Read the model definition and answer for the solid it produces. Units are mm, in the model's axes. A direction names the side the tool comes from. Coordinates: 2 decimals unless noted, no trailing zeros. Order: outer loops, then holes, each group sorted by start corner. A loop starts at its lowest first (then second) coordinate and runs counter-clockwise, first axis right, second up. Notation, with made-up numbers: (8.25, 27.5) - (58.25, 27.5) arc R8 ccw to (58.25, 34.5) - close; hole circle Ø8 at (38.5, -27.75). An arc over 180 degrees is marked (long way). Use one line per item in the form item = value.
```python
from build123d import *

# Parameters (mm, degrees)
F0_R     = 26.745197
F1_DEPTH = 50.8
F2_R     = 33.58545
F3_DEPTH = 101.6
F4_DEPTH = 50.8
F5_DEPTH = 25.4
F6_W     = 15.942245
F6_H     = 27.044877
F7_DEPTH = 152.4


with BuildPart() as f1:
    # F0 (on Top) → F1 (new body)
    with BuildSketch(Plane.XY):
        with Locations((-60.452543, 36.618207)):
            Circle(F0_R)
    extrude(amount=F1_DEPTH)

    # F2 (on Top) → F3 (join)
    with BuildSketch(Plane.XY):
        with Locations((-27.838308, 13.809561)):
            Circle(F2_R)
    extrude(amount=F3_DEPTH)

    # F0 (on Top) → F4 (join)
    with BuildSketch(Plane.XY):
        with Locations((-60.452543, 36.618207)):
            Circle(F0_R)
    extrude(amount=F4_DEPTH)

    # F0 (on Top) → F5 (join)
    with BuildSketch(Plane.XY):
        with Locations((-60.452543, 36.618207)):
            Circle(F0_R)
    extrude(amount=-F5_DEPTH)

    # F6 (on Top) → F7 (join)
    with BuildSketch(Plane.XY):
        with Locations((-24.767418, 13.522438)):
            Rectangle(F6_W, F6_H)
    extrude(amount=-F7_DEPTH)


solid = f1.part
```
(1) Section D-D, the plane y = -8 is taken. Write down the section's boundary in (x, z).
Answer list:
outline = (-53.38, 0) - (-2.3, 0) - (-2.3, 101.6) - (-53.38, 101.6) - close
(2) Section B-B, the plane x = -21 is taken. Write down the section's boundary in (y, z), then the cut area to 3 significant figures.
Answer list:
outline = (-19.07, 0) - (0, 0) - (0, -152.4) - (27.04, -152.4) - (27.04, 0) - (46.69, 0) - (46.69, 101.6) - (-19.07, 101.6) - close
area = 10,800 mm2
(3) Given pin 1 Ø12 at (x, y) = (-33.5, -6.5) entering from -Z; pin 2 Ø1 at (x, y) = (-69.5, 15.5) entering from -Z; pin 3 Ø13.5 at (y, z) = (19.5, -85) entering from -X, each flat-ended and moving along its own axis, determine where each tip first touches the part or whether it passes through.
Answer list:
pin_1 = 0
pin_2 = -25.4
pin_3 = -32.74
(4) Section A-A, the plane z = -68 is taken. Write down the section's boundary in (x, y).
Answer list:
outline = (-32.74, 0) - (-16.8, 0) - (-16.8, 27.04) - (-32.74, 27.04) - close
(5) Straight lines are drawn through the part: L1, parallel to Z at x = -79.5, y = 23; L2, parallel to Z at x = -2, y = 18; L3, parallel to X at y = 10.5, z = -88. For each, find the intervals that lie inside material, in ascending order.
Answer list:
L1 = -25.4 to 50.8
L2 = 0 to 101.6
L3 = -32.74 to -16.8
(6) Which of the six approach directions +Z, -Z, +X, -X, +Y, -Y give full straight-line access (tool end or side, diameter ignored) to faces 1 (the flat face through (-25, 27.045, -75)), 2 (the flat face through (-25, 0, -75)), 3 (the flat face through (-32.739, 13, -75)), 4 (the flat face through (-61, 37, -25.4))?
Answer list:
face_1 = -Z, +X, +Y
face_2 = -Z, +X, -X, -Y
face_3 = -Z, +Y, -Y
face_4 = -Z, -X, +Y, -Y
(7) Section C-C, the plane y = 2.5 is taken. Write down the section's boundary in (x, z), then the cut area to 3 significant figures.
Answer list:
outline = (-59.46, 0) - (-32.74, 0) - (-32.74, -152.4) - (-16.8, -152.4) - (-16.8, 0) - (3.79, 0) - (3.79, 101.6) - (-59.46, 101.6) - close
area = 8,860 mm2
